Answer from the drawing. Dimensions are ordinates in mm from the lowest x, y and z of the part. A direction names the side the tool comes from. Coordinates: 2 decimals unless noted, no trailing zeros. Order: outer loops, then holes, each group sorted by start corner. A loop starts at its lowest first (then second) coordinate and runs counter-clockwise, first axis right, second up. Notation, with made-up numbers: (-31, 65) -> (15, 65) arc R23 cw to (15, 89) -> close; hole circle Ø11 at (40.5, 78). An arc over 180 degrees is marked (long way). Use CSV: the item, a comma, the result in double quotes.
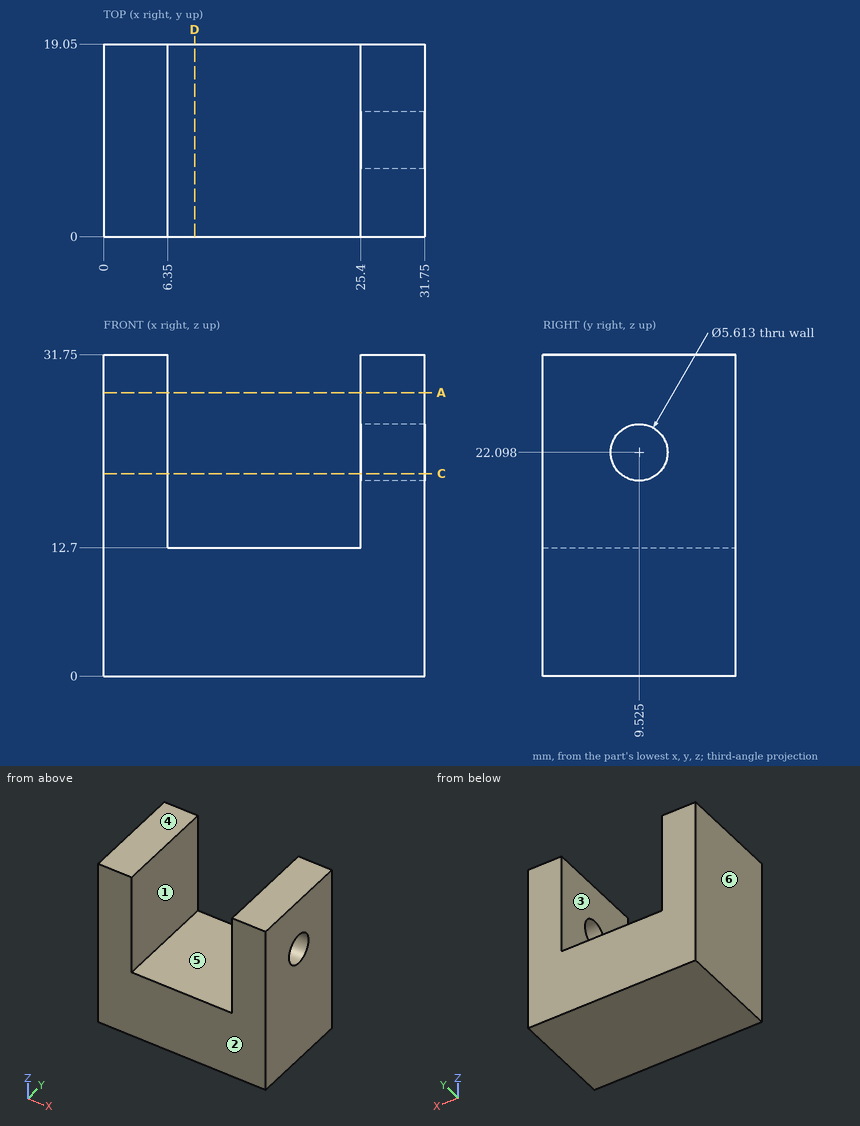
Item 1: Find section C-C, the plane z = 20. Give the vertices of the cut face in (x, y).
Return value:
outline,"(0, 0) -> (6.35, 0) -> (6.35, 19.05) -> (0, 19.05) -> close; (25.4, 0) -> (31.75, 0) -> (31.75, 7.66) -> (25.4, 7.66) -> close; (25.4, 11.39) -> (31.75, 11.39) -> (31.75, 19.05) -> (25.4, 19.05) -> close"
Item 2: A tool of negligible diameter and unlimited length cuts with its end or side. For the marked faces 1 and 2, from which of +Z, -Z, +X, -X, +Y, -Y can it reach the whole face along a straight path? Write none if from no direction.
Return value:
face 1,"+Z, +Y, -Y"
face 2,"+Z, -Z, +X, -X, -Y"
Item 3: Find section A-A, the plane z = 28. Give the vertices of the cut face in (x, y).
Return value:
outline,"(0, 0) -> (6.35, 0) -> (6.35, 19.05) -> (0, 19.05) -> close; (25.4, 0) -> (31.75, 0) -> (31.75, 19.05) -> (25.4, 19.05) -> close"
Item 4: Straight lines are drawn through the part: line 1 along X through (y, z) = (16, 25); line 2 along Y through (x, z) = (30, 22); line 3 along Z through (x, y) = (25, 10). For each, find the intervals that lie inside material, in ascending order.
Return value:
line 1,"x = 0 to 6.35, 25.4 to 31.75"
line 2,"y = 0 to 6.72, 12.33 to 19.05"
line 3,"z = 0 to 12.7"
Item 5: Find section D-D, the plane x = 9. Give the vertices of the cut face in (y, z), then the cut area to 3 significant figures.
Return value:
outline,"(0, 0) -> (19.05, 0) -> (19.05, 12.7) -> (0, 12.7) -> close"
area,"242 mm^2"
Item 6: Each of these flat-tipped pins is pushed along its axis until it touches: P1, Ø10, axis at x = 24, z = 3.5, coming from the -Y side; P2, Ø4.5, axis at y = 9.525, z = 22.098, coming from the +X side; P3, Ø5.5, axis at x = 16.5, y = 5.5, coming from the +Z side. Where does it stop, or does it pass through?
Return value:
P1,"stops at y = 0"
P2,"stops at x = 6.35"
P3,"stops at z = 12.7"
Item 7: The mould has two halves that part along X. Classify the marked faces 3, 4, 5 and 6: +X half, -X half, draft (parallel to the pull), parting line (faces both ways), or undercut.
Return value:
face 3,"undercut"
face 4,"draft"
face 5,"undercut"
face 6,"-X half"
